```python
from build123d import *

# Parameters (mm, degrees)
SKETCH3_W           = 50.8
SKETCH3_H           = 50.8
BOSS_EXTRUDE1_DEPTH = 29.996194
CUT_EXTRUDE1_DEPTH  = 65.230613146
CIRPATTERN1_COUNT   = 4
SKETCH8_W           = 12.7
SKETCH8_H           = 12.7
CUT_EXTRUDE2_DEPTH  = 44.00537756
CUT_EXTRUDE3_START  = -20.21
CUT_EXTRUDE3_DEPTH  = 84.434853552
SKETCH10_W          = 2.032
SKETCH10_H          = 12.7
CUT_EXTRUDE4_DEPTH  = 21.76
CIRPATTERN2_COUNT   = 4
SKETCH11_W          = 6.35
SKETCH11_H          = 6.35
CUT_EXTRUDE5_DEPTH  = 41.659838908


with BuildPart() as part:
    # Sketch3 → Boss-Extrude1 (new body)
    with BuildSketch(Plane(origin=(0, 0, 0), x_dir=(0, 0, -1), z_dir=(1, 0, 0))):
        Rectangle(SKETCH3_W, SKETCH3_H)
    extrude(amount=BOSS_EXTRUDE1_DEPTH)

    # Sketch4 → Cut-Loft1 section 0
    with BuildSketch(Plane(origin=(12.7, 0, 0), x_dir=(0, 0, -1), z_dir=(1, 0, 0))):
        with BuildLine():
            Line((-3.507611845, 3.507611845), (3.507611845, 3.507611845))
            Line((3.507611845, 3.507611845), (3.507611845, -3.507611845))
            Line((3.507611845, -3.507611845), (-3.507611845, -3.507611845))
            Line((-3.507611845, -3.507611845), (-3.507611845, 3.507611845))
        make_face()
    # Sketch5 → Cut-Loft1 section 1
    with BuildSketch(Plane(origin=(29.996194078, 0, 0), x_dir=(0, 0, -1), z_dir=(1, 0, 0))):
        with BuildLine():
            Line((-20.803805922, 20.803805922), (20.803805922, 20.803805922))
            Line((20.803805922, 20.803805922), (20.803805922, -20.803805922))
            Line((20.803805922, -20.803805922), (-20.803805922, -20.803805922))
            Line((-20.803805922, -20.803805922), (-20.803805922, 20.803805922))
        make_face()
    loft(mode=Mode.SUBTRACT)

    # Sketch6 → Cut-Extrude1 (cut, through all)
    with BuildSketch(Plane(origin=(0, 25.4, 0), x_dir=(1, 0, 0), z_dir=(0, 1, 0))):
        Polygon((25.4, -25.4), (0, 0), (0, -25.4), align=None)
    cut_extrude1 = extrude(amount=-CUT_EXTRUDE1_DEPTH, mode=Mode.SUBTRACT)

    # CirPattern1: Cut-Extrude1 ×4 about axis
    cirpattern1_axis = Axis((0, 0, 0), (1, 0, 0))
    for i in range(1, CIRPATTERN1_COUNT):
        add(cut_extrude1.rotate(cirpattern1_axis, i * 360 / CIRPATTERN1_COUNT), mode=Mode.SUBTRACT)

    # Sketch8 → Cut-Extrude2 (cut, through all)
    with BuildSketch(Plane(origin=(6.35, 0, 0), x_dir=(0, 0, -1), z_dir=(1, 0, 0))):
        Rectangle(SKETCH8_W, SKETCH8_H)
    extrude(amount=-CUT_EXTRUDE2_DEPTH, mode=Mode.SUBTRACT)

    # Sketch9 → Cut-Extrude3 (cut)
    with BuildSketch(Plane(origin=(31.142405514, 0, 26.921685137), x_dir=(0.7071067811865474, 0, -0.7071067811865477), z_dir=(0.7071067811865477, 0, 0.7071067811865474)).offset(CUT_EXTRUDE3_START)):
        Polygon((-1.016, 5.08), (-1.016, 6.35), (1.016, 6.35), (1.016, 5.08), (3.5155, 5.08), (3.5155, -5.08), (1.016, -5.08), (1.016, -6.35), (-1.016, -6.35), (-1.016, -5.08), (-3.5155, -5.08), (-3.5155, 5.08), align=None)
    cut_extrude3 = extrude(amount=CUT_EXTRUDE3_DEPTH, mode=Mode.SUBTRACT)

    # Sketch10 → Cut-Extrude4 (cut)
    with BuildSketch(Plane(origin=(31.142405514, 0, 26.921685137), x_dir=(0.7071067811865474, 0, -0.7071067811865477), z_dir=(0.7071067811865477, 0, 0.7071067811865474))):
        Rectangle(SKETCH10_W, SKETCH10_H)
    cut_extrude4 = extrude(amount=-CUT_EXTRUDE4_DEPTH, mode=Mode.SUBTRACT)

    # CirPattern2: Cut-Extrude3, Cut-Extrude4 ×4 about axis
    cirpattern2_axis = Axis((0, 0, 0), (1, 0, 0))
    add([cut_extrude3.rotate(cirpattern2_axis, i * 360 / CIRPATTERN2_COUNT) for i in range(1, CIRPATTERN2_COUNT)], mode=Mode.SUBTRACT)
    add([cut_extrude4.rotate(cirpattern2_axis, i * 360 / CIRPATTERN2_COUNT) for i in range(1, CIRPATTERN2_COUNT)], mode=Mode.SUBTRACT)

    # Sketch11 → Cut-Extrude5 (cut, through all)
    with BuildSketch(Plane(origin=(25.4, 0, 0), x_dir=(0, 0, -1), z_dir=(1, 0, 0))):
        with Locations((22.225, 22.225)):
            Rectangle(SKETCH11_W, SKETCH11_H)
        with Locations((22.225, -22.225)):
            Rectangle(SKETCH11_W, SKETCH11_H)
        with Locations((-22.225, -22.225)):
            Rectangle(SKETCH11_W, SKETCH11_H)
        with Locations((-22.225, 22.225)):
            Rectangle(SKETCH11_W, SKETCH11_H)
    extrude(amount=-CUT_EXTRUDE5_DEPTH, mode=Mode.SUBTRACT)


solid = part.part
```
Model file for the job. Use its own axes, mm. A direction names the side the tool comes from. Coordinates: 2 decimals unless noted, no trailing zeros. Order: outer loops, then holes, each group sorted by start corner. A loop starts at its lowest first (then second) coordinate and runs counter-clockwise, first axis right, second up. Notation, with made-up numbers: (23.25, 17.5) -> (57.25, 17.5) arc R25 ccw to (57.25, 33.5) -> close; hole circle Ø4 at (57, 6). An arc over 180 degrees is marked (long way). Answer as a JSON object with one key per item and string values. Group by question number.
1) Cut at B-B, the plane x = 23. Count the separate pieces of the cut face and the enclosed holes in it, then the cut area to 3 significant figures.
2) Cut at A-A, the plane x = 8. Write the cut outline in (y, z), then the cut area to 3 significant figures.
3) Flat gauge pins, fed straight in: pin 1 (6 mm diameter, centred on x = 21, z = -17, fed in from +Y); pin 2 (3 mm diameter, centred on x = 19.5, y = -8.5, fed in from +Z); pin 3 (7 mm diameter, centred on y = 22, z = 21.5, fed in from -X). Where does each tip first touch, or does it go through?
4) Which spindle directions (+Z, -Z, +X, -X, +Y, -Y) get a long thin tool onto all of the face, cutting with end or side? Do faces 4 (the face through (23, 19.05, -21)), 5 (the face through (6.35, 0, 0)), 6 (the face through (24, -19.05, 21)), 7 (the face through (23, -18, -6.35)). Say none if no direction does.
5) Drill centre lines: L1, parallel to Y at x = 26.5, z = 20.5; L2, parallel to Z at x = 19, y = 14; L3, parallel to X at y = -12.5, z = -6. Where is each one in solid material? Low to high.
6) Pull direction Y, two halves, no side cores. Call faces 1 (the face through (15.447, 14.036, -0.071)), 2 (the face through (21, 20, -5.08)), 3 (the face through (15.447, 0.071, 14.036)): +Y half, -Y half, draft (parallel to the pull), parting line (faces both ways), or undercut.
Check values:
{
 "1": {"separate pieces": "4", "enclosed holes": "0", "area": "888 mm²"},
 "2": {"outline": "(-8, -8) -> (8, -8) -> (8, 8) -> (-8, 8) -> close", "area": "256 mm²"},
 "3": {"pin 1": "stops at y = 24", "pin 2": "stops at z = 21", "pin 3": "stops at x = 19.5"},
 "4": {"face 4": "-Z, -X, +Y", "face 5": "+Z, -Z, -X, +Y, -Y", "face 6": "+Z, -X, -Y", "face 7": "none"},
 "5": {"L1": "y = -25.4 to -5.08, 5.08 to 25.4", "L2": "z = -19 to -6.35, 6.35 to 19", "L3": "x = 12.5 to 15.28, 18.16 to 21.69"},
 "6": {"face 1": "+Y half", "face 2": "draft", "face 3": "undercut"}
}
